Could you check a few things on this model? Use its own coordinates, in mm. Give positions to 0.01 mm unless a question says otherwise; leave off trailing zeros. Loops run counter-clockwise (first coordinate to the right, second up) from the corner with the lowest first, then second, coordinate; pieces in that order, holes last. Notation, with made-up numbers: (82, -15) - (101, -15) arc R19 ccw to (101, 14) - close; hole circle Ø6 at (-18, 52). An arc over 180 degrees is marked (long way). Write each question's results on one line, items separated by ' | '. Start each with the question number.
1) If I drill on probe 1 along Z at (x, y) = (73, 0.25), over which ranges is the centre line in solid material (lowest first)? Write a range as [from, to].
2) I want a section at A-A, the plane y = 0.15. Write out the boundary of the cut face in (x, z), and give its area (3 significant figures).
3) I want a section at B-B, the plane x = -89. Write out the boundary of the cut face in (y, z), and give its area (3 significant figures).
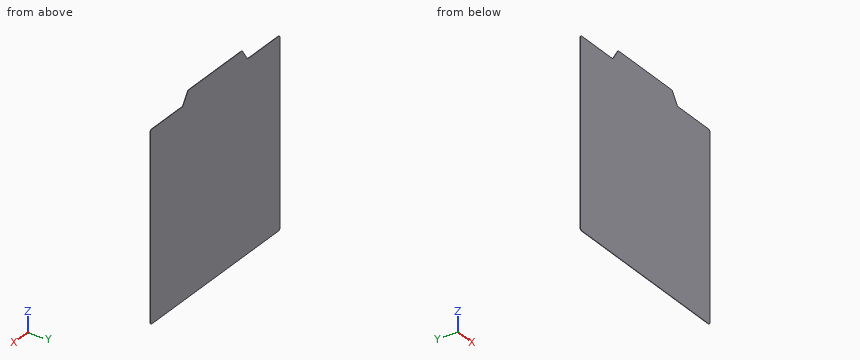
from build123d import *

# Parameters (mm, degrees)
AUFSATZ_LINEAR_AUSTRAGEN1_DEPTH = 0.5
BOSS_EXTRUDE1_DEPTH             = 0.5
FILLET1_R                       = 2


with BuildPart() as part:
    # Skizze1 → Aufsatz-Linear austragen1 (new body)
    with BuildSketch(Plane(origin=(0, 0, 0), x_dir=(1, 0, 0), z_dir=(0, 1, 0))):
        with BuildLine():
            Line((-117, -120), (117, -120))
            ThreePointArc((117, -120), (119.121320344, -119.121320344), (120, -117))
            Line((120, -117), (120, 117))
            ThreePointArc((120, 117), (119.121320344, 119.121320344), (117, 120))
            Line((117, 120), (-117, 120))
            ThreePointArc((-117, 120), (-119.121320344, 119.121320344), (-120, 117))
            Line((-120, 117), (-120, -117))
            ThreePointArc((-120, -117), (-119.121320344, -119.121320344), (-117, -120))
        make_face()
    extrude(amount=AUFSATZ_LINEAR_AUSTRAGEN1_DEPTH)

    # Sketch1 → Boss-Extrude1 (add)
    with BuildSketch(Plane(origin=(0, 0.5, 0), x_dir=(1, 0, 0), z_dir=(0, 1, 0))):
        Polygon((-60, -120), (-50, -135), (50, -135), (60, -120), align=None)
    extrude(amount=-BOSS_EXTRUDE1_DEPTH)

    # Fillet1
    fillet1_edges = [part.edges().sort_by_distance(p)[0] for p in [
        (-60, 0.25, 120),
        (60, 0.25, 120),
        (50, 0.25, 135),
        (-50, 0.25, 135),
    ]]
    fillet(fillet1_edges, radius=FILLET1_R)


solid = part.part
Answers:
1) probe 1: z = [-120, 120]
2) outline: (-120, -117) arc R3 ccw to (-117, -120) - (117, -120) arc R3 ccw to (120, -117) - (120, 117) arc R3 ccw to (117, 120) - (61.07, 120) arc R2 cw to (59.41, 120.89) - (50.59, 134.11) arc R2 ccw to (48.93, 135) - (-48.93, 135) arc R2 ccw to (-50.59, 134.11) - (-59.41, 120.89) arc R2 cw to (-61.07, 120) - (-117, 120) arc R3 ccw to (-120, 117) - close | area: 59,200 mm2
3) outline: (0, -120) - (0.5, -120) - (0.5, 120) - (0, 120) - close | area: 120 mm2
